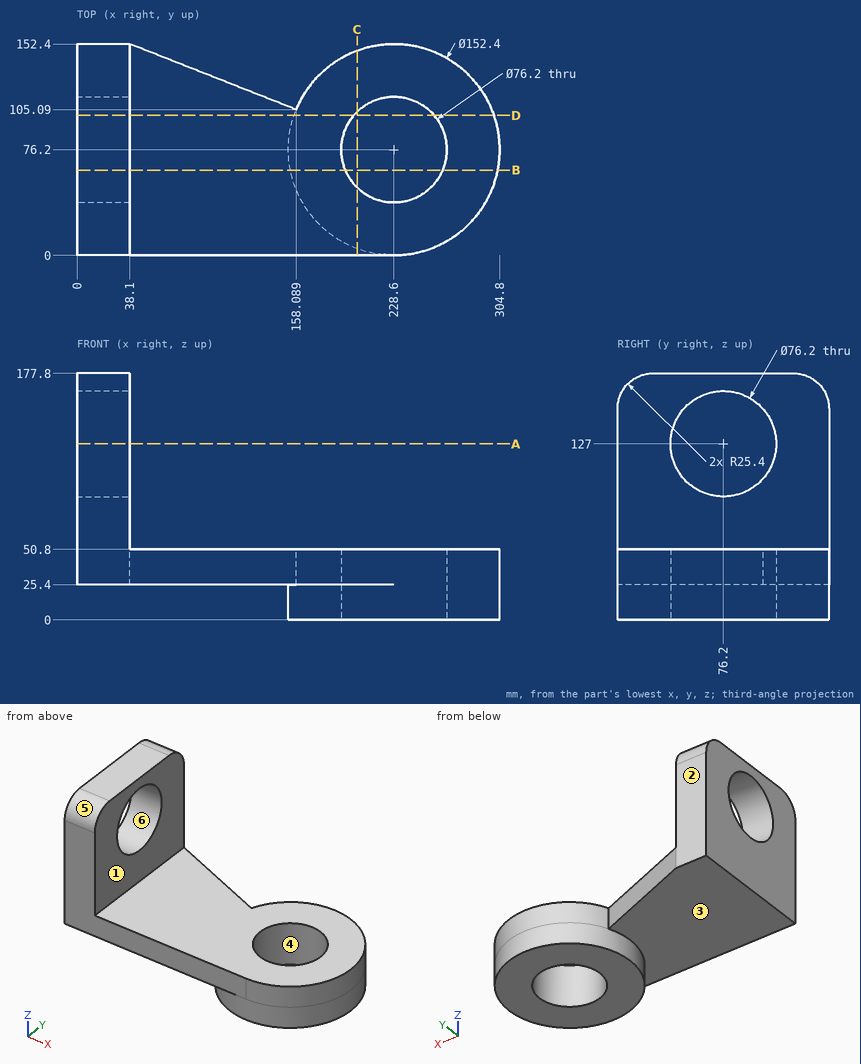
Check sheet for the drawn part. Datum: minimum x, y, z corner. Units: mm. A direction names the side the tool comes from. Give positions to 0.01 mm unless a question says otherwise; leave off trailing zeros. Order: outer loops, then holes, each group sorted by start corner. A loop starts at its lowest first (then second) coordinate and runs counter-clockwise, first axis right, second up. Notation, with made-up numbers: (22.5, 33.5) - (65.5, 33.5) arc R30 ccw to (65.5, 71.5) - close; hole circle Ø1 at (35, -14.5). An arc over 180 degrees is marked (long way). Answer as a JSON object with one key per item and string values.
(1) Cross-section at C-C (x = 202). Record the cut outline in (y, z), then the cut area to 3 significant figures.
Report:
{"outline": "(0, 25.4) - (4.79, 25.4) - (4.79, 0) - (48.92, 0) - (48.92, 50.8) - (0, 50.8) - close; (103.48, 0) - (147.61, 0) - (147.61, 50.8) - (103.48, 50.8) - close", "area": "4,610 mm^2"}
(2) Draft check along Y on the marked faces 3, 4, 5 and 6. Enter one of: released by +Y, released by -Y, zero draft, split by the parting line, or undercut.
Report:
{"face 3": "zero draft", "face 4": "undercut", "face 5": "released by -Y", "face 6": "undercut"}
(3) Cross-section at A-A (z = 127). Record the cut outline in (x, y), then the cut area to 3 significant figures.
Report:
{"outline": "(0, 0) - (38.1, 0) - (38.1, 38.1) - (0, 38.1) - close; (0, 114.3) - (38.1, 114.3) - (38.1, 152.4) - (0, 152.4) - close", "area": "2,900 mm^2"}
(4) Cross-section at B-B (y = 61.5). Record the cut outline in (x, z).
Report:
{"outline": "(0, 25.4) - (153.83, 25.4) - (153.83, 0) - (193.45, 0) - (193.45, 50.8) - (38.1, 50.8) - (38.1, 91.85) - (0, 91.85) - close; (0, 162.15) - (38.1, 162.15) - (38.1, 177.8) - (0, 177.8) - close; (263.75, 0) - (303.37, 0) - (303.37, 50.8) - (263.75, 50.8) - close"}
(5) Material ranges on line 1 (X direction, y = 76, z = 15); line 2 (Z direction, x = 22, y = 76); line 3 (Z direction, x = 226.5, y = 135), recorded low to high.
Report:
{"line 1": "152.4 to 190.5, 266.7 to 304.8", "line 2": "25.4 to 88.9, 165.1 to 177.8", "line 3": "0 to 50.8"}
(6) Cross-section at D-D (y = 101). Record the cut outline in (x, z).
Report:
{"outline": "(0, 25.4) - (156.55, 25.4) - (156.55, 0) - (199.68, 0) - (199.68, 50.8) - (38.1, 50.8) - (38.1, 98.08) - (0, 98.08) - close; (0, 155.92) - (38.1, 155.92) - (38.1, 177.8) - (0, 177.8) - close; (257.52, 0) - (300.65, 0) - (300.65, 50.8) - (257.52, 50.8) - close"}
(7) Tool access check on the marked faces 1 and 2. Record the directions out of +Z, -Z, +X, -X, +Y, -Y that give a thin tool (end or side, any length) a straight path to the whole face; none if there is none.
Report:
{"face 1": "+Z, +X, +Y, -Y", "face 2": "+Z, -Z, +X, -X, +Y"}
(8) Depth check by flat-ended pin: pin 1 Ø8 at (y, z) = (135.5, 71) entering from +X; pin 2 Ø3 at (x, y) = (148, 79.5) entering from +Z; pin 3 Ø12 at (x, z) = (189.5, 39.5) entering from +Y. Enter the tip coordinate at first touch or a pass-through.
Report:
{"pin 1": "x = 38.1", "pin 2": "z = 50.8", "pin 3": "y = 144.84"}
